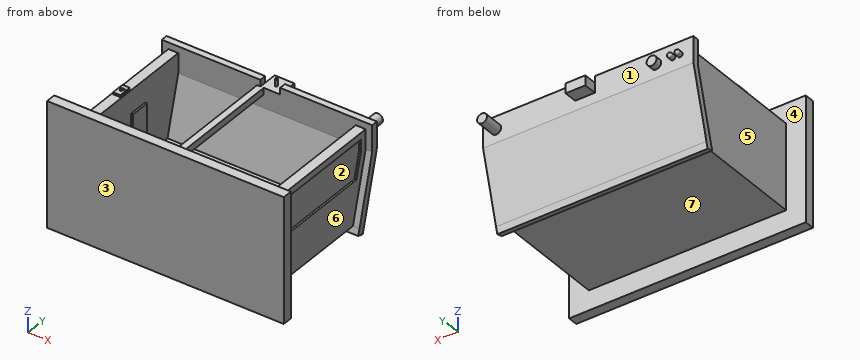
```python
from build123d import *

# Parameters (mm, degrees)
SALIENTE_EXTRUIR11_DEPTH      = 200
CORTAR_EXTRUIR10_DEPTH        = 300
SALIENTE_EXTRUIR12_DEPTH      = 10
SALIENTE_EXTRUIR12_DEPTH_BACK = 310
CROQUIS30_W                   = 360
CROQUIS30_H                   = 190
SALIENTE_EXTRUIR13_DEPTH      = 15
CORTAR_EXTRUIR11_DEPTH        = 15
CROQUIS32_W                   = 5
CROQUIS32_H                   = 55
SALIENTE_EXTRUIR14_DEPTH      = 180
CROQUIS35_W                   = 11
CROQUIS35_H                   = 20
SALIENTE_EXTRUIR15_DEPTH      = 3
CORTAR_EXTRUIR12_DEPTH        = 1
CROQUIS40_W                   = 150
CROQUIS40_H                   = 10
SALIENTE_EXTRUIR16_DEPTH      = 10
CROQUIS41_W                   = 10
CROQUIS41_H                   = 10
SALIENTE_EXTRUIR17_DEPTH      = 190
CROQUIS42_W                   = 50
CROQUIS42_H                   = 30
SALIENTE_EXTRUIR18_DEPTH      = 3
CROQUIS43_W                   = 30
CROQUIS43_H                   = 10
CORTAR_EXTRUIR13_DEPTH        = 10
CROQUIS44_R                   = 7.5
SALIENTE_EXTRUIR19_DEPTH      = 30
CROQUIS45_W                   = 30
CROQUIS45_H                   = 15
SALIENTE_EXTRUIR20_DEPTH      = 20
CROQUIS47_R                   = 2
SALIENTE_EXTRUIR21_DEPTH      = 10
CORTAR_EXTRUIR14_START        = -10
CROQUIS49_R                   = 2
CORTAR_EXTRUIR14_DEPTH        = 10
CROQUIS50_R                   = 2
SALIENTE_EXTRUIR22_DEPTH      = 10
CROQUIS52_R                   = 3.75
SALIENTE_EXTRUIR29_DEPTH      = 10
REDONDEO6_R                   = 3.7
CROQUIS53_R                   = 7.5
SALIENTE_EXTRUIR30_DEPTH      = 10


with BuildPart() as part:
    # Croquis4 → Saliente-Extruir11 (new body)
    with BuildSketch(Plane(origin=(0, 0, 0), x_dir=(1, 0, 0), z_dir=(0, 1, 0))):
        Polygon((-150, 65), (150, 65), (150, -65), (135, -65), (135, 50), (-135, 50), (-135, -65), (-150, -65), align=None)
    extrude(amount=SALIENTE_EXTRUIR11_DEPTH)

    # Croquis28 → Cortar-Extruir10 (cut)
    with BuildSketch(Plane.ZY.offset(150)):
        Polygon((-65, 173.205080757), (35, 200), (-65, 200), align=None)
    extrude(amount=-CORTAR_EXTRUIR10_DEPTH, mode=Mode.SUBTRACT)

    # Croquis29 → Saliente-Extruir12 (add, two sides: drawn at the far end of the back side and taken through both)
    with BuildSketch(Plane.ZY.offset(150).offset(-SALIENTE_EXTRUIR12_DEPTH_BACK)):
        Polygon((-65, 173.205080757), (35, 200), (65, 200), (75, 200), (75, 210), (35, 210), (-67.5, 182.535207776), (-77.159258263, 179.947017325), (-74.571067812, 170.287759062), align=None)
    extrude(amount=SALIENTE_EXTRUIR12_DEPTH + SALIENTE_EXTRUIR12_DEPTH_BACK)

    # Croquis30 → Saliente-Extruir13 (add)
    with BuildSketch(Plane.XZ):
        Rectangle(CROQUIS30_W, CROQUIS30_H)
    extrude(amount=SALIENTE_EXTRUIR13_DEPTH)

    # Croquis31 → Cortar-Extruir11 (cut)
    with BuildSketch(Plane(origin=(150, 0, 0), x_dir=(0, 0, -1), z_dir=(1, 0, 0))):
        Polygon((-55, 190), (-55, 10), (0, 10), (0, 180.269016461), (-36.316524976, 190), align=None)
    extrude(amount=-CORTAR_EXTRUIR11_DEPTH, mode=Mode.SUBTRACT)

    # Croquis32 → Saliente-Extruir14 (add)
    with BuildSketch(Plane(origin=(0, 10, 0), x_dir=(1, 0, 0), z_dir=(0, 1, 0))):
        with Locations((144.5, -27.5)):
            Rectangle(CROQUIS32_W, CROQUIS32_H)
    extrude(amount=SALIENTE_EXTRUIR14_DEPTH)

    # Croquis35 → Saliente-Extruir15 (add)
    with BuildSketch(Plane.XY.offset(65)):
        with Locations((-142.5, 90)):
            Rectangle(CROQUIS35_W, CROQUIS35_H)
    extrude(amount=SALIENTE_EXTRUIR15_DEPTH)

    # Croquis36 → Cortar-Extruir12 (cut)
    with BuildSketch(Plane.XY.offset(68)):
        with BuildLine():
            Line((-143.875, 87.38156986), (-144.5, 88.464101615))
            ThreePointArc((-144.5, 88.464101615), (-142.5, 89), (-140.5, 88.464101615))
            Line((-140.5, 88.464101615), (-141.125, 87.38156986))
            ThreePointArc((-141.125, 87.38156986), (-142.5, 87.75), (-143.875, 87.38156986))
        make_face()
        with BuildLine():
            Line((-139.875, 89.54663337), (-139.25, 90.629165125))
            ThreePointArc((-139.25, 90.629165125), (-142.5, 91.5), (-145.75, 90.629165125))
            Line((-145.75, 90.629165125), (-145.125, 89.54663337))
            ThreePointArc((-145.125, 89.54663337), (-142.5, 90.25), (-139.875, 89.54663337))
        make_face()
        with BuildLine():
            Line((-146.375, 91.711696879), (-147, 92.794228634))
            ThreePointArc((-147, 92.794228634), (-142.5, 94), (-138, 92.794228634))
            Line((-138, 92.794228634), (-138.625, 91.711696879))
            ThreePointArc((-138.625, 91.711696879), (-142.5, 92.75), (-146.375, 91.711696879))
        make_face()
    extrude(amount=-CORTAR_EXTRUIR12_DEPTH, mode=Mode.SUBTRACT)

    # Croquis40 → Saliente-Extruir16 (add)
    with BuildSketch(Plane(origin=(0, 0, 0), x_dir=(1, 0, 0), z_dir=(0, 1, 0))):
        with Locations((60, -60)):
            Rectangle(CROQUIS40_W, CROQUIS40_H)
    extrude(amount=SALIENTE_EXTRUIR16_DEPTH)

    # Croquis41 → Saliente-Extruir17 (add)
    with BuildSketch(Plane(origin=(0, 10, 0), x_dir=(1, 0, 0), z_dir=(0, 1, 0))):
        with Locations((-10, -60)):
            Rectangle(CROQUIS41_W, CROQUIS41_H)
    extrude(amount=SALIENTE_EXTRUIR17_DEPTH)

    # Croquis42 → Saliente-Extruir18 (add)
    with BuildSketch(Plane(origin=(-135, 0, 0), x_dir=(0, 0, -1), z_dir=(1, 0, 0))):
        with Locations((-5, 115)):
            Rectangle(CROQUIS42_W, CROQUIS42_H)
    extrude(amount=SALIENTE_EXTRUIR18_DEPTH)

    # Croquis43 → Cortar-Extruir13 (cut)
    with BuildSketch(Plane(origin=(0, 210, 0), x_dir=(1, 0, 0), z_dir=(0, 1, 0))):
        with Locations((5, -70)):
            Rectangle(CROQUIS43_W, CROQUIS43_H)
    extrude(amount=-CORTAR_EXTRUIR13_DEPTH, mode=Mode.SUBTRACT)

    # Croquis44 → Saliente-Extruir19 (add)
    with BuildSketch(Plane(origin=(0, 210, 0), x_dir=(1, 0, 0), z_dir=(0, 1, 0))):
        with Locations(Location((140, -55, 0), (0, 0, 90))):
            Circle(CROQUIS44_R)
    extrude(amount=SALIENTE_EXTRUIR19_DEPTH)

    # Croquis45 → Saliente-Extruir20 (add)
    with BuildSketch(Plane(origin=(0, 210, 0), x_dir=(1, 0, 0), z_dir=(0, 1, 0))):
        with Locations((5, -57.5)):
            Rectangle(CROQUIS45_W, CROQUIS45_H)
    extrude(amount=SALIENTE_EXTRUIR20_DEPTH)

    # Croquis47 → Saliente-Extruir21 (add)
    with BuildSketch(Plane.XY.offset(65)):
        with Locations(Location((5, 215, 0), (0, 0, 180))):
            Circle(CROQUIS47_R)
    extrude(amount=SALIENTE_EXTRUIR21_DEPTH)

    # Croquis49 → Cortar-Extruir14 (cut)
    with BuildSketch(Plane.XY.offset(75).offset(CORTAR_EXTRUIR14_START)):
        with Locations((5, 215)):
            Circle(CROQUIS49_R)
    extrude(amount=CORTAR_EXTRUIR14_DEPTH, mode=Mode.SUBTRACT)

    # Croquis50 → Saliente-Extruir22 (add)
    with BuildSketch(Plane.XY.offset(65)):
        with Locations(Location((5, 213, 0), (0, 0, 180))):
            Circle(CROQUIS50_R)
    extrude(amount=SALIENTE_EXTRUIR22_DEPTH)

    # Croquis52 → Saliente-Extruir29 (add)
    with BuildSketch(Plane(origin=(0, 210, 0), x_dir=(1, 0, 0), z_dir=(0, 1, 0))):
        with Locations(Location((-140, -55, 0), (0, 0, 90))):
            Circle(CROQUIS52_R)
        with Locations(Location((-128.75988107, -55, 0), (0, 0, 90))):
            Circle(CROQUIS52_R)
    extrude(amount=SALIENTE_EXTRUIR29_DEPTH)

    # Redondeo6
    redondeo6_edges = [part.edges().sort_by_distance(p)[0] for p in [
        (-140, 220, 58.75),
        (-128.75988107, 220, 58.75),
    ]]
    fillet(redondeo6_edges, radius=REDONDEO6_R)

    # Croquis53 → Saliente-Extruir30 (add)
    with BuildSketch(Plane(origin=(0, 210, 0), x_dir=(1, 0, 0), z_dir=(0, 1, 0))):
        with Locations(Location((-103.450024464, -55, 0), (0, 0, 90))):
            Circle(CROQUIS53_R)
    extrude(amount=SALIENTE_EXTRUIR30_DEPTH)


solid = part.part
```
The listing builds one solid part. Answer for the finished solid, in the listing's coordinates (mm). Face numbers are marked on the shaded views. A direction names the side the tool comes from. Coordinates: 2 decimals unless noted, no trailing zeros. Loops run counter-clockwise (first coordinate to the right, second up) from the corner with the lowest first, then second, coordinate; pieces in that order, holes last. Notation, with made-up numbers: (-1, 84.25) -> (53, 84.25) arc R19 ccw to (53, 117.25) -> close; hole circle Ø10 at (68.25, 45). An arc over 180 degrees is marked (long way). Return JSON: item names as keys, results as strings. Group by question number.
(1) A cutting plane is placed at D-D on x = -29. Write down the section's boundary in (y, z).
(2) A cutting plane is placed at B-B on x = 74.5. Write down the section's boundary in (y, z).
(3) Find the intervals of material crossed by probe 1 along X at (y, z) = (27, 62.5); probe 2 along X at (y, z) = (136, 11.5); probe 3 along X at (y, z) = (73, -11), in increasing order. Write a range as from..to.
(4) A cutting plane is placed at A-A on y = 30. Write down the section's boundary in (x, z), and give its area (3 significant figures).
(5) Given pin 1 Ø1.5 at (x, y) = (-51, 41) entering from -Z; pin 2 Ø2.5 at (x, z) = (-133.5, 12) entering from +Y; pin 3 Ø12 at (y, z) = (119, 67) entering from +X, each flat-ended and moving along its own axis, determine where each tip first touches the part or whether it passes through.
(6) Which of the six approach directions +Z, -Z, +X, -X, +Y, -Y give full straight-line access (tool end or side, diameter ignored) to the marked faces 1, 2 and 3?
(7) Determine the mould class of the marked faces 4, 5, 6 and 7 for opening direction X: released by +X, released by -X, zero draft, split by the parting line, or undercut.
(8) A cutting plane is placed at C-C on y = 124. Write down the section's boundary in (x, z).
The answers:
{
 "1": {"outline": "(-15, -95) -> (0, -95) -> (0, -65) -> (173.21, -65) -> (170.29, -74.57) -> (179.95, -77.16) -> (210, 35) -> (210, 75) -> (200, 75) -> (200, 35) -> (177.22, -50) -> (0, -50) -> (0, 95) -> (-15, 95) -> close"},
 "2": {"outline": "(-15, -95) -> (0, -95) -> (0, -65) -> (173.21, -65) -> (170.29, -74.57) -> (179.95, -77.16) -> (210, 35) -> (210, 75) -> (200, 75) -> (200, 35) -> (177.22, -50) -> (0, -50) -> (0, 55) -> (10, 55) -> (10, 65) -> (0, 65) -> (0, 95) -> (-15, 95) -> close"},
 "3": {"probe 1": "x = -150..-135, -15..-5, 135..150", "probe 2": "x = -150..-135, 142..147", "probe 3": "x = -150..-135, 135..150"},
 "4": {"outline": "(-150, -65) -> (150, -65) -> (150, 0) -> (147, 0) -> (147, 55) -> (150, 55) -> (150, 65) -> (135, 65) -> (135, 55) -> (142, 55) -> (142, 0) -> (135, 0) -> (135, -50) -> (-135, -50) -> (-135, 65) -> (-150, 65) -> close; (-15, 55) -> (-5, 55) -> (-5, 65) -> (-15, 65) -> close", "area": "7,500 mm^2"},
 "5": {"pin 1": "stops at z = -65", "pin 2": "stops at y = 204.17", "pin 3": "stops at x = 150"},
 "6": {"face 1": "+Y", "face 2": "+X", "face 3": "+Z, -Z, +X, -X, -Y"},
 "7": {"face 4": "undercut", "face 5": "released by -X", "face 6": "released by +X", "face 7": "zero draft"},
 "8": {"outline": "(-150, -65) -> (150, -65) -> (150, 0) -> (147, 0) -> (147, 55) -> (150, 55) -> (150, 65) -> (135, 65) -> (135, 55) -> (142, 55) -> (142, 0) -> (135, 0) -> (135, -50) -> (-135, -50) -> (-135, -20) -> (-132, -20) -> (-132, 30) -> (-135, 30) -> (-135, 65) -> (-150, 65) -> close; (-15, 55) -> (-5, 55) -> (-5, 65) -> (-15, 65) -> close"}
}
